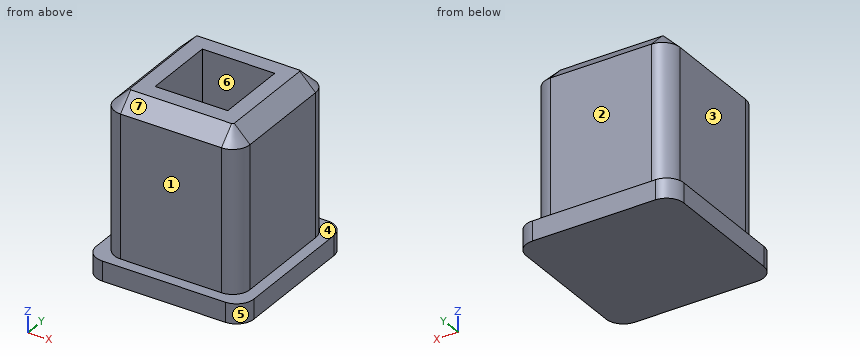
from build123d import *

# Parameters (mm, degrees)
F0_W     = 20
F0_H     = 20
F1_DEPTH = 2.5
F2_W     = 17.2
F2_H     = 17.2
F3_DEPTH = 20
F4_R     = 2.2
F5_W     = 9.2
F5_H     = 9.2
F6_DEPTH = 15.2
F7_SIZE  = 2


with BuildPart() as f1:
    # F0 (on Top) → F1 (new body)
    with BuildSketch(Plane.XY):
        Rectangle(F0_W, F0_H)
    extrude(amount=F1_DEPTH)

    # F2 (on face) → F3 (join)
    with BuildSketch(Plane.XY.offset(2.5)):
        Rectangle(F2_W, F2_H)
    extrude(amount=F3_DEPTH)

    # F4
    f4_edges = [f1.edges().sort_by_distance(p)[0] for p in [
        (-8.6, -8.6, 12.5),
        (-8.6, 8.6, 12.5),
        (8.6, 8.6, 12.5),
        (8.6, -8.6, 12.5),
        (10, -10, 1.25),
        (10, 10, 1.25),
        (-10, -10, 1.25),
        (-10, 10, 1.25),
    ]]
    fillet(f4_edges, radius=F4_R)

    # F5 (on face) → F6 (cut)
    with BuildSketch(Plane.XY.offset(22.5)):
        Rectangle(F5_W, F5_H)
    extrude(amount=-F6_DEPTH, mode=Mode.SUBTRACT)

    # F7
    f7_edges = [f1.edges().sort_by_distance(p)[0] for p in [
        (0, 8.6, 22.5),
    ]]
    chamfer(f7_edges, length=F7_SIZE)


solid = f1.part
Part model, mm, in its own coordinate system. Face numbers are marked on the shaded views. A direction names the side the tool comes from. Round coordinates to 2 decimals unless told otherwise and drop trailing zeros. Order: outer loops, then holes, each group sorted by start corner. A loop starts at its lowest first (then second) coordinate and runs counter-clockwise, first axis right, second up. Notation, with made-up numbers: (45, 82.25) -> (76, 82.25) arc R11 cw to (76, 89.25) -> close; hole circle Ø9 at (-39, -2.75). An arc over 180 degrees is marked (long way). Put each result on its own line as item: value.
Q1. Wall check: line 1 (Y direction, x = 3.75, z = 20); line 2 (X direction, y = -6.25, z = 17). Give the ranges that are in metal, low to high. Write a range as [from, to].
From the geometry:
line 1: y = [-8.6, -4.6], [4.6, 8.6]
line 2: x = [-8.6, 8.6]
Q2. Pull direction X, two halves, no side cores. Call the marked faces 5, 6 and 7: pulls with the +X half, pulls with the -X half, needs draft (parallel to the pull), parting line crosses it, or undercut.
From the geometry:
face 5: pulls with the +X half
face 6: undercut
face 7: needs draft
Q3. Band-saw the part on C-C (z = 6). Give the cut face in (x, y).
From the geometry:
outline: (-8.6, -6.4) arc R2.2 ccw to (-6.4, -8.6) -> (6.4, -8.6) arc R2.2 ccw to (8.6, -6.4) -> (8.6, 6.4) arc R2.2 ccw to (6.4, 8.6) -> (-6.4, 8.6) arc R2.2 ccw to (-8.6, 6.4) -> close
Q4. Tool access for the marked faces 1, 2, 3 and 4: list every direction of +Z, -Z, +X, -X, +Y, -Y with a clear straight run to the whole face (end or side of a thin tool).
From the geometry:
face 1: +Z, +X, -X, -Y
face 2: +Z, +X, -X, +Y
face 3: +Z, -X, +Y, -Y
face 4: +Z
Q5. Band-saw the part on D-D (x = -5.5). Give the cut face in (y, z).
From the geometry:
outline: (-10, 0) -> (10, 0) -> (10, 2.5) -> (8.6, 2.5) -> (8.6, 20.5) -> (6.6, 22.5) -> (-6.6, 22.5) -> (-8.6, 20.5) -> (-8.6, 2.5) -> (-10, 2.5) -> close
Q6. Pin check, flat tips, straight feed: pin 1 Ø6.5 at (y, z) = (0, 15.5) entering from +X; pin 2 Ø6 at (x, y) = (-3.5, -5.5) entering from -Z; pin 3 Ø4.5 at (x, z) = (-0.5, 14.5) entering from +Y; pin 4 Ø7.5 at (x, z) = (1.5, 14.5) entering from -Y. Stop position of each tip, or through.
From the geometry:
pin 1: stops at x = 8.6
pin 2: stops at z = 0
pin 3: stops at y = 8.6
pin 4: stops at y = -8.6
Q7. Band-saw the part on A-A (z = 10). Give the cut face in (x, y), and give its area (3 significant figures).
From the geometry:
outline: (-8.6, -6.4) arc R2.2 ccw to (-6.4, -8.6) -> (6.4, -8.6) arc R2.2 ccw to (8.6, -6.4) -> (8.6, 6.4) arc R2.2 ccw to (6.4, 8.6) -> (-6.4, 8.6) arc R2.2 ccw to (-8.6, 6.4) -> close; hole (-4.6, -4.6) -> (4.6, -4.6) -> (4.6, 4.6) -> (-4.6, 4.6) -> close
area: 207 mm2
Q8. Band-saw the part on B-B (y = 0). Give the cut face in (x, z), and give its area (3 significant figures).
From the geometry:
outline: (-10, 0) -> (10, 0) -> (10, 2.5) -> (8.6, 2.5) -> (8.6, 20.5) -> (6.6, 22.5) -> (4.6, 22.5) -> (4.6, 7.3) -> (-4.6, 7.3) -> (-4.6, 22.5) -> (-6.6, 22.5) -> (-8.6, 20.5) -> (-8.6, 2.5) -> (-10, 2.5) -> close
area: 250 mm2
